Build history of the part. All positions in model axes, mm. Round coordinates to 2 decimals unless told otherwise and drop trailing zeros. Write each loop counter-clockwise with the first axis right and the second up, starting at its lowest first coordinate (ties: lowest second). Pieces come first, ordered by that corner, then holes.
Item 1: Band-saw the part on B-B, the plane y = 140. Write the cut outline in (x, z).
Item 2: Wall check: probe 1 along Y at (x, z) = (255, 3.75); probe 2 along Y at (x, z) = (206, 2.75). Give the ranges that are in metal, low to high.
Item 3: Band-saw the part on A-A, the plane z = 8.25. Write the cut outline in (x, y).
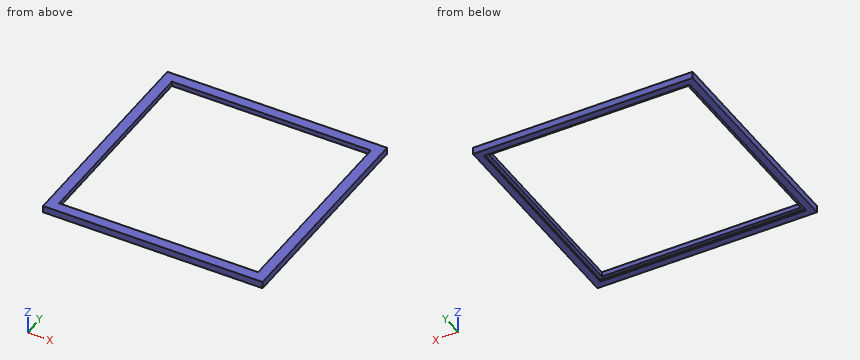
```python
from build123d import *

# Parameters (mm, degrees)
CROQUIS1_W              = 320
CROQUIS1_H              = 320
CROQUIS1_W_2            = 290
CROQUIS1_H_2            = 290
SALIENTE_EXTRUIR1_DEPTH = 10
CROQUIS2_W              = 300
CROQUIS2_H              = 300
CORTAR_EXTRUIR1_DEPTH   = 3


with BuildPart() as part:
    # Croquis1 → Saliente-Extruir1 (new body)
    with BuildSketch(Plane.XY):
        with Locations((150, 150)):
            Rectangle(CROQUIS1_W, CROQUIS1_H)
        with Locations((150, 150)):
            Rectangle(CROQUIS1_W_2, CROQUIS1_H_2, mode=Mode.SUBTRACT)
    extrude(amount=SALIENTE_EXTRUIR1_DEPTH)

    # Croquis2 → Cortar-Extruir1 (cut)
    with BuildSketch(Plane(origin=(0, 0, 0), x_dir=(-1, 0, 0), z_dir=(0, 0, -1))):
        with Locations((-150, 150)):
            Rectangle(CROQUIS2_W, CROQUIS2_H)
    extrude(amount=-CORTAR_EXTRUIR1_DEPTH, mode=Mode.SUBTRACT)


solid = part.part
```
Results:
1. outline: (-10, 0) - (0, 0) - (0, 3) - (5, 3) - (5, 10) - (-10, 10) - close; (295, 3) - (300, 3) - (300, 0) - (310, 0) - (310, 10) - (295, 10) - close
2. probe 1: y = -10 to 5, 295 to 310
2. probe 2: y = -10 to 0, 300 to 310
3. outline: (-10, -10) - (310, -10) - (310, 310) - (-10, 310) - close; hole (5, 5) - (295, 5) - (295, 295) - (5, 295) - close
